Solid Edge part; units mm, degrees
sketch "Sketch1" plane through (0, 0, 0) normal (0, 0, 1) x (1, 0, 0)
  circle A0 centre (0, 0) radius 35.3568
  circle A1 centre (0, 0) radius 40.4368
extrude "Protrusion1" add sketch "Sketch1" along normal blind 12.7
sketch "Sketch2" plane through (0, 0, 12.7) normal (0, 0, 1) x (0, 1, 0)
  circle A0 centre (0, 0) radius 50.8
extrude "ExtrudedProtrusion_2" add sketch "Sketch2" against normal blind 5.08
sketch "Sketch3" plane through (0, 0, 12.7) normal (0, 0, 1) x (0, 1, 0)
  circle A0 centre (0, 0) radius 48.0568
  circle A1 centre (0, 0) radius 50.8
extrude "ExtrudedProtrusion_3" add sketch "Sketch3" against normal blind 20.32
sketch "Sketch4" plane through (0, 0, 0) normal (0, 0, 1) x (1, 0, 0)
  circle A0 centre (0, 0) radius 35.3568
extrude "Cutout1" cut sketch "Sketch4" along normal up to next
sketch "Sketch5" plane through (0, 0, -7.62) normal (0, 0, -1) x (-1, 0, 0)
  circle A0 centre (0, 49.4284) radius 0.9525
extrude "ExtrudedCutout_2" cut sketch "Sketch5" against normal blind 6.35
pattern_circular "Pattern_1" count 16 over 360 about axis through (0, 0, 0) along (0, 0, -1) of "ExtrudedCutout_2"
For this review, take the finished solid that the model builds, in its own axes (mm). A direction names the side the tool comes from. Give positions to 0.01 mm unless a question says otherwise; leave off trailing zeros. Write each loop counter-clockwise with the first axis right and the second up, starting at its lowest first coordinate (ties: lowest second). Pieces come first, ordered by that corner, then holes.
Item 1: Insertion check: P1, Ø1.5, axis at x = -34.95, y = 34.95, coming from the -Z side; P2, Ø5, axis at y = -29.5, z = -0.5, coming from the +X side; P3, Ø3, axis at x = 36.5, z = 1.5, coming from the -Y side. Each pin has a flat end and moves straight along its axis. Give the tip position at first contact, or say it passes through.
Item 2: Machinability: for faces 1 (the face through (-8.766, 39.475, 3.757)), 2 (the face through (-35, -11, 12.7)), which of the approach directions +Z, -Z, +X, -X, +Y, -Y give a long, thin tool a straight path to every point of the face, cutting with its end or side? Answer none if there is none.
Item 3: Take a section at C-C (x = -13). Give the boundary of the cut face in (y, z), and give its area (3 significant figures).
Item 4: The part is to be moulded in two halves that separate along X. For faces 3 (the face through (49.592, -11.012, 2.682)), 4 (the face through (41, -26, -7.62)), 5 (the face through (46.914, -10.418, 0.107)), say which applies: +X half, -X half, draft (parallel to the pull), parting line (faces both ways), or undercut.
Item 5: Take a section at B-B (y = -4). Give the boundary of the cut face in (x, z).
Item 6: Take a section at D-D (y = -39). Give the boundary of the cut face in (x, z), and give its area (3 significant figures).
Item 7: Take a section at A-A (z = 6). Give the boundary of the cut face in (x, y), and give its area (3 significant figures).
Item 8: Wall thickness on probe 1 along Y at (x, z) = (0, -4.5); probe 2 along X at (y, z) = (-4.5, 0.5); probe 3 along X at (y, z) = (2, 2.5): over which ranges is each line inside the solid? List them lowest first.
Established:
1. P1: stops at z = -1.27
1. P2: stops at x = 43.03
1. P3: stops at y = -36.82
2. face 1: -Z
2. face 2: +Z, +X, -X, +Y, -Y
3. outline: (-49.11, -7.62) - (-46.27, -7.62) - (-46.27, 7.62) - (-38.29, 7.62) - (-38.29, 0) - (-32.88, 0) - (-32.88, 12.7) - (-49.11, 12.7) - close; (32.88, 0) - (38.29, 0) - (38.29, 7.62) - (46.27, 7.62) - (46.27, -7.62) - (49.11, -7.62) - (49.11, 12.7) - (32.88, 12.7) - close
3. area: 334 mm2
4. face 3: parting line
4. face 4: draft
4. face 5: undercut
5. outline: (-50.64, -7.62) - (-47.89, -7.62) - (-47.89, 7.62) - (-40.24, 7.62) - (-40.24, 0) - (-35.13, 0) - (-35.13, 12.7) - (-50.64, 12.7) - close; (35.13, 0) - (40.24, 0) - (40.24, 7.62) - (47.89, 7.62) - (47.89, -7.62) - (50.64, -7.62) - (50.64, 12.7) - (35.13, 12.7) - close
6. outline: (-32.55, -7.62) - (-28.08, -7.62) - (-28.08, 7.62) - (-10.68, 7.62) - (-10.68, 0) - (10.68, 0) - (10.68, 7.62) - (28.08, 7.62) - (28.08, -7.62) - (32.55, -7.62) - (32.55, 12.7) - (-32.55, 12.7) - close
6. area: 630 mm2
7. outline: circle Ø101.6 at (0, 0); circle Ø80.87 at (0, 0); hole circle Ø96.11 at (0, 0); hole circle Ø70.71 at (0, 0)
7. area: 2,060 mm2
8. probe 1: y = -50.8 to -50.38, -48.48 to -48.06, 48.06 to 48.48, 50.38 to 50.8
8. probe 2: x = -50.6 to -47.85, -40.19 to -35.07, 35.07 to 40.19, 47.85 to 50.6
8. probe 3: x = -50.76 to -48.02, -40.39 to -35.3, 35.3 to 40.39, 48.02 to 50.76
